```python
from build123d import *

# Parameters (mm, degrees)
SKETCH1_W           = 30
SKETCH1_H           = 25
BOSS_EXTRUDE1_DEPTH = 3
SKETCH2_R           = 1.6
CUT_EXTRUDE2_DEPTH  = 10
SKETCH3_W           = 8
SKETCH3_H           = 3
BOSS_EXTRUDE2_DEPTH = 5


with BuildPart() as part:
    # Sketch1 → Boss-Extrude1 (new body)
    with BuildSketch(Plane(origin=(0, 0, 0), x_dir=(1, 0, 0), z_dir=(0, 1, 0))):
        with Locations((-7.290640394, 2.155172414)):
            Rectangle(SKETCH1_W, SKETCH1_H)
    extrude(amount=BOSS_EXTRUDE1_DEPTH)

    # Sketch2 → Cut-Extrude2 (cut)
    with BuildSketch(Plane(origin=(0, 3, 0), x_dir=(1, 0, 0), z_dir=(0, 1, 0))):
        with Locations(Location((-15.790640394, 2.155172414, 0), (0, 0, 270))):
            Circle(SKETCH2_R)
        with Locations(Location((1.209359606, 2.155172414, 0), (0, 0, 270))):
            Circle(SKETCH2_R)
    extrude(amount=-CUT_EXTRUDE2_DEPTH, mode=Mode.SUBTRACT)

    # Sketch3 → Boss-Extrude2 (add)
    with BuildSketch(Plane(origin=(0, 3, 0), x_dir=(1, 0, 0), z_dir=(0, 1, 0))):
        with Locations((-7.290640394, 13.155172414)):
            Rectangle(SKETCH3_W, SKETCH3_H)
    extrude(amount=BOSS_EXTRUDE2_DEPTH)


solid = part.part
```
Source: CAD feature listing. Evaluate the final solid. Frame: model axes, mm. A direction names the side the tool comes from. Round coordinates to 2 decimals unless told otherwise and drop trailing zeros. Loops run counter-clockwise (first coordinate to the right, second up) from the corner with the lowest first, then second, coordinate; pieces in that order, holes last.
1. Mould query, pull axis X, two halves, no side actions, for faces 1 (the cylindrical face through (0.236, 1.521, -3.425)), 2 (the cylindrical face through (-16.764, 1.521, -3.425)), 3 (the flat face through (-8, 1, 10.345)), 4 (the flat face through (-11.291, 5, -13)). Classes: released by +X, released by -X, zero draft, split by the parting line, or undercut.
2. Section query B-B on z = -12.75. Output: boundary loops of the cut face in (x, y).
3. Ray query, L1, parallel to Y at x = -17, z = -0.5; L2, parallel to Z at x = -9.25, y = 3.75; L3, parallel to X at y = 7, z = -13. Return the intervals inside material, ascending.
4. Section query C-C on y = 2.5. Output: boundary loops of the cut face in (x, z), and give its area (3 significant figures).
5. Access query for faces 5 (the flat face through (-7, 8, -13)), 6 (the flat face through (-7, 5, -11.655)), 7 (the flat face through (-3.291, 5, -13)). Directions: +Z, -Z, +X, -X, +Y, -Y. A direction counts if a zero-diameter tool reaches every point of the face in a straight line with its end or side. Return the directions, or none.
6. Contact query for flat-ended pins moving along their axis: pin 1 (4 mm diameter, centred on y = 6.5, z = 4.5, fed in from +X); pin 2 (2.5 mm diameter, centred on x = -8.5, y = 5, fed in from +Z); pin 3 (0.9 mm diameter, centred on y = 6.5, z = -13, fed in from +X); pin 4 (5 mm diameter, centred on x = -15.79, z = -2.16, fed in from +Y). Output: stop coordinate, or through.
7. Section query A-A on x = -16.5. Output: boundary loops of the cut face in (y, z), and give its area (3 significant figures).
8. Section query D-D on x = -6. Output: boundary loops of the cut face in (y, z), and give its area (3 significant figures).
Answers below:
1. face 1: undercut
1. face 2: undercut
1. face 3: zero draft
1. face 4: released by -X
2. outline: (-22.29, 0) - (7.71, 0) - (7.71, 3) - (-3.29, 3) - (-3.29, 8) - (-11.29, 8) - (-11.29, 3) - (-22.29, 3) - close
3. L1: y = 0 to 3
3. L2: z = -14.66 to -11.66
3. L3: x = -11.29 to -3.29
4. outline: (-22.29, -14.66) - (7.71, -14.66) - (7.71, 10.34) - (-22.29, 10.34) - close; hole circle Ø3.2 at (-15.79, -2.16); hole circle Ø3.2 at (1.21, -2.16)
4. area: 734 mm2
5. face 5: +Z, -Z, +X, -X, +Y
5. face 6: +Z, +X, -X, +Y
5. face 7: +Z, -Z, +X, +Y
6. pin 1: passes through
6. pin 2: stops at z = -11.66
6. pin 3: stops at x = -3.29
6. pin 4: stops at y = 3
7. outline: (0, -14.66) - (3, -14.66) - (3, -3.59) - (0, -3.59) - close; (0, -0.72) - (3, -0.72) - (3, 10.34) - (0, 10.34) - close
7. area: 66.4 mm2
8. outline: (0, -14.66) - (8, -14.66) - (8, -11.66) - (3, -11.66) - (3, 10.34) - (0, 10.34) - close
8. area: 90.0 mm2
